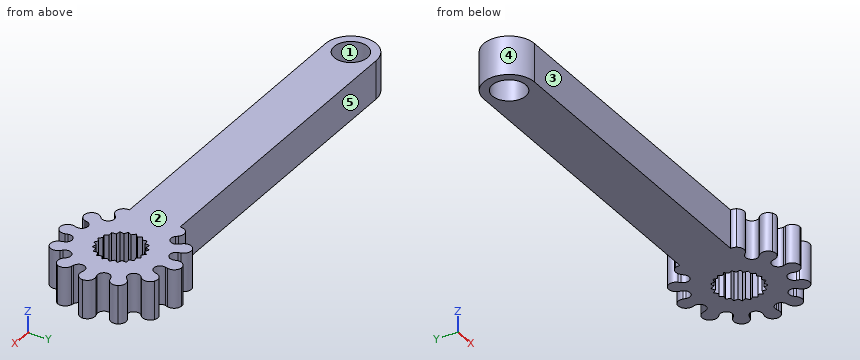
```python
from build123d import *

# Parameters (mm, degrees)
SKETCH1_R           = 1.65
BOSS_EXTRUDE1_DEPTH = 3.8
CUT_EXTRUDE1_DEPTH  = 26.02878343
CIRPATTERN1_COUNT   = 12
SKETCH3_W           = 5.990659071
SKETCH3_H           = 5
BOSS_EXTRUDE2_DEPTH = 3.8
SKETCH4_R           = 2.1
CUT_EXTRUDE2_DEPTH  = 26.02878343
CUT_EXTRUDE3_DEPTH  = 10


with BuildPart() as part:
    # Sketch1 → Boss-Extrude1 (new body)
    with BuildSketch(Plane.XY):
        with BuildLine():
            Line((-18, 2.5), (12.545643943, 2.5))
            ThreePointArc((12.545643943, 2.5), (24, 0), (12.545643943, -2.5))
            Line((12.545643943, -2.5), (-18, -2.5))
            ThreePointArc((-18, -2.5), (-20.5, 0), (-18, 2.5))
        make_face()
        with Locations(Location((-18, 0, 0), (0, 0, 180))):
            Circle(SKETCH1_R, mode=Mode.SUBTRACT)
    extrude(amount=BOSS_EXTRUDE1_DEPTH)

    # Sketch2 → Cut-Extrude1 (cut, through all)
    with BuildSketch(Plane.XY.offset(3.8)):
        with BuildLine():
            ThreePointArc((21, 5.196152423), (19.633748274, 6.097231567), (18, 6))
            ThreePointArc((18, 6), (19.552914271, 5.795554958), (21, 5.196152423))
        make_face()
        with BuildLine():
            ThreePointArc((18, 6), (18.589879661, 5.706078038), (18.72, 5.06))
            Line((18.72, 5.06), (18.654523502, 4.81))
            ThreePointArc((18.654523502, 4.81), (19.09327028, 4.062778187), (19.840492093, 4.501524965))
            Line((19.840492093, 4.501524965), (19.906461709, 4.742088543))
            ThreePointArc((19.906461709, 4.742088543), (20.342188248, 5.236548367), (21, 5.196152423))
            ThreePointArc((21, 5.196152423), (19.552914271, 5.795554958), (18, 6))
        make_face()
    cut_extrude1 = extrude(amount=-CUT_EXTRUDE1_DEPTH, mode=Mode.SUBTRACT)

    # CirPattern1: Cut-Extrude1 ×12 about axis
    cirpattern1_axis = Axis((18, 0, 0), (0, 0, 1))
    for i in range(1, CIRPATTERN1_COUNT):
        add(cut_extrude1.rotate(cirpattern1_axis, i * 360 / CIRPATTERN1_COUNT), mode=Mode.SUBTRACT)

    # Sketch3 → Boss-Extrude2 (add)
    with BuildSketch(Plane.XY.offset(3.8)):
        with Locations((13.282390893, 0)):
            Rectangle(SKETCH3_W, SKETCH3_H)
    extrude(amount=-BOSS_EXTRUDE2_DEPTH)

    # Sketch4 → Cut-Extrude2 (cut, through all)
    with BuildSketch(Plane.XY.offset(3.8)):
        with Locations((18, 0)):
            Circle(SKETCH4_R)
    extrude(amount=-CUT_EXTRUDE2_DEPTH, mode=Mode.SUBTRACT)

    # Sketch5 → Cut-Extrude3 (cut)
    with BuildSketch(Plane.XY.offset(3.8)):
        Polygon((20.006712152, 0.618955846), (20.373196658, 0.357683687), (20.1, 0), (20.373191307, -0.35771919), (20.006702892, -0.618985866), (20.162317494, -1.041337148), (19.735101426, -1.182972122), (19.759312282, -1.63242773), (19.309328584, -1.641846113), (19.199984453, -2.078469945), (18.767216151, -1.954834872), (18.53403274, -2.339830984), (18.156933197, -2.094127974), (17.820629874, -2.393287772), (17.532706039, -2.047348616), (17.123164831, -2.234090438), (16.95, -1.818653348), (16.50361044, -1.876384365), (16.460591069, -1.428362749), (16.017016829, -1.351953307), (16.107965377, -0.911155852), (15.706619975, -0.707395264), (15.923455265, -0.312988759), (15.6, 1.7952e-05), (15.923455265, 0.312988759), (15.706630558, 0.707429573), (16.107965377, 0.911155852), (16.017037054, 1.351982972), (16.460591069, 1.428362749), (16.503638511, 1.876406751), (16.95, 1.818653348), (17.123198253, 2.234103555), (17.532706039, 2.047348616), (17.820665677, 2.393290455), (18.156933197, 2.094127974), (18.534067743, 2.339822994), (18.767216151, 1.954834872), (19.200015547, 2.078451993), (19.309328584, 1.641846113), (19.759336703, 1.632401411), (19.735101426, 1.182972122), (20.162333072, 1.0413048), align=None)
    extrude(amount=-CUT_EXTRUDE3_DEPTH, mode=Mode.SUBTRACT)


solid = part.part
```
Can you work these out from the model? Positions are in its coordinate system, mm. Face numbers are marked on the shaded views. A direction names the side the tool comes from. Coordinates: 2 decimals unless noted, no trailing zeros. Loops run counter-clockwise (first coordinate to the right, second up) from the corner with the lowest first, then second, coordinate; pieces in that order, holes last. Notation, with made-up numbers: M 24.5,15.5 L 43.5,15.5 A22 ccw 43.5,50.5 Z; hole C 33,-16.5 d6. An arc over 180 degrees is marked long. Put each result on its own line as item: value. Start each with the question number.
(1) Imagine slicing it at A-A on z = 2.6. Give the number of separate pieces and of enclosed holes in the cut face, and give its area (3 significant figures).
(2) Imagine slicing it at B-B on x = 4. List the corners of the cut face in (y, z) for me, and give its area (3 significant figures).
(3) We'd pull the mould along Y, two halves only. Please class the marked faces 1, 2 and 3: +Y half, -Y half, draft (parallel to the pull), parting line (faces both ways), or undercut.
(4) Which directions (+Z, -Z, +X, -X, +Y, -Y) give clear straight access to the entire face, cutting with the end or side of a thin tool? Please do the marked faces 4 and 5.
(5) I need wall thicknesses on probe 1 along Y at (x, z) = (-18, 1.55); probe 2 along X at (y, z) = (-4.5, 0.8); probe 3 along X at (y, z) = (-0.5, 2.9). Which ranges of each line are inside material? Lowest first, please.
(6) Will these pins go through, and if not, where does the flat tip stop? pin 1 Ø2 at (y, z) = (-1.5, 1.5) entering from +X; pin 2 Ø1 at (x, y) = (-12.5, -3.5) entering from -Z.
Worked answers:
1. separate pieces: 1
1. enclosed holes: 2
1. area: 225 mm2
2. outline: M -2.5,0 L 2.5,0 L 2.5,3.8 L -2.5,3.8 Z
2. area: 19.0 mm2
3. face 1: undercut
3. face 2: draft
3. face 3: -Y half
4. face 4: +Z, -Z, -X
4. face 5: +Z, -Z, -X, +Y
5. probe 1: y = -2.5 to -1.65, 1.65 to 2.5
5. probe 2: x = 14.63 to 16.16, 17.35 to 18.65, 19.84 to 21.37
5. probe 3: x = -20.45 to -19.57, -16.43 to 15.82, 20.17 to 23.8
6. pin 1: stops at x = 23.8
6. pin 2: passes through
